For this review, take the finished solid that the model builds, in its own axes (mm). A direction names the side the tool comes from. Give positions to 0.01 mm unless a question says otherwise; leave off trailing zeros. Order: outer loops, then holes, each group sorted by start corner. A loop starts at its lowest first (then second) coordinate and runs counter-clockwise, first axis right, second up. Notation, with made-up numbers: (76, 13) -> (115, 13) arc R19 ccw to (115, 31) -> close; hole circle Ø4 at (30.25, -6). An arc over 180 degrees is marked (long way). Use CSV: the item, a comma, the result in double quotes. Start each with the question number.
```python
from build123d import *

# Parameters (mm, degrees)
SKETCH2_R          = 3.96875
CUT_EXTRUDE1_DEPTH = 6.35
CUT_EXTRUDE2_START = -41.402
CUT_EXTRUDE2_DEPTH = 31.75
SKETCH3_4_R        = 14.605
CUT_EXTRUDE3_DEPTH = 9.652


with BuildPart() as part:
    # Sketch1 → Revolve1 (revolve)
    with BuildSketch(Plane(origin=(0, 0, 0), x_dir=(1, 0, 0), z_dir=(0, 1, 0))):
        Polygon((-20.701, -12.7), (-20.701, -29.845), (-13.081, -29.845), (-13.081, -32.385), (5.969, -32.385), (5.969, -40.005), (7.239, -40.005), (7.239, -23.495), (20.701, -23.495), (20.701, -12.7), align=None)
    revolve(axis=Axis((-34.012862719, 0, 0), (1, 0, 0)))

    # Sketch2 → Cut-Extrude1 (cut)
    with BuildSketch(Plane(origin=(-20.701, 0, 0), x_dir=(0, 0, -1), z_dir=(1, 0, 0))):
        with Locations((22.225, 0)):
            Circle(SKETCH2_R)
        with Locations((-11.1125, -19.247414599)):
            Circle(SKETCH2_R)
        with Locations((-11.1125, 19.247414599)):
            Circle(SKETCH2_R)
    extrude(amount=CUT_EXTRUDE1_DEPTH, mode=Mode.SUBTRACT)

    # Sketch3 → Cut-Extrude2 (cut)
    with BuildSketch(Plane(origin=(20.701, 0, 0), x_dir=(0, 0, -1), z_dir=(1, 0, 0)).offset(CUT_EXTRUDE2_START)):
        with BuildLine():
            Line((-13.214999101, -6.218506553), (-10.722964654, -6.805000296))
            ThreePointArc((-10.722964654, -6.805000296), (-11.491303566, -5.407397003), (-12.078417757, -3.924515829))
            Line((-12.078417757, -3.924515829), (-13.214999101, -6.218506553))
        make_face()
        with BuildLine():
            Line((-14.346305297, -2.7367041), (-12.078417757, -3.924515829))
            ThreePointArc((-12.078417757, -3.924515829), (-12.475048084, -2.379742695), (-12.674939451, -0.797439598))
            Line((-12.674939451, -0.797439598), (-14.346305297, -2.7367041))
        make_face()
        with BuildLine():
            Line((-14.576180369, 0.917055538), (-12.674939451, -0.797439598))
            ThreePointArc((-12.674939451, -0.797439598), (-12.674939451, 0.797439598), (-12.475048084, 2.379742695))
            Line((-12.475048084, 2.379742695), (-14.576180369, 0.917055538))
        make_face()
        with BuildLine():
            Line((-13.89018042, 4.513193203), (-12.475048084, 2.379742695))
            ThreePointArc((-12.475048084, 2.379742695), (-12.078417757, 3.924515829), (-11.491303566, 5.407397003))
            Line((-11.491303566, 5.407397003), (-13.89018042, 4.513193203))
        make_face()
        with BuildLine():
            Line((-12.331409352, 7.825750341), (-11.491303566, 5.407397003))
            ThreePointArc((-11.491303566, 5.407397003), (-10.722964654, 6.805000296), (-9.785518183, 8.09528467))
            Line((-9.785518183, 8.09528467), (-12.331409352, 7.825750341))
        make_face()
        with BuildLine():
            Line((-9.997810482, 10.646586803), (-9.785518183, 8.09528467))
            ThreePointArc((-9.785518183, 8.09528467), (-8.693748245, 9.257901568), (-7.464872704, 10.274515829))
            Line((-7.464872704, 10.274515829), (-9.997810482, 10.646586803))
        make_face()
        with BuildLine():
            Line((-7.03601241, 12.798459062), (-7.464872704, 10.274515829))
            ThreePointArc((-7.464872704, 10.274515829), (-6.118271661, 11.129094837), (-4.675181819, 11.808161371))
            Line((-4.675181819, 11.808161371), (-7.03601241, 12.798459062))
        make_face()
        with BuildLine():
            Line((-3.632115802, 14.146157068), (-4.675181819, 11.808161371))
            ThreePointArc((-4.675181819, 11.808161371), (-3.158361567, 12.301006146), (-1.591732066, 12.599856707))
            Line((-1.591732066, 12.599856707), (-3.632115802, 14.146157068))
        make_face()
        with BuildLine():
            ThreePointArc((-1.591732066, 12.599856707), (0, 12.7), (1.591732066, 12.599856707))
            Line((1.591732066, 12.599856707), (0, 14.605))
            Line((0, 14.605), (-1.591732066, 12.599856707))
        make_face()
        with BuildLine():
            ThreePointArc((1.591732066, 12.599856707), (3.158361567, 12.301006146), (4.675181819, 11.808161371))
            Line((4.675181819, 11.808161371), (3.632115802, 14.146157068))
            Line((3.632115802, 14.146157068), (1.591732066, 12.599856707))
        make_face()
        with BuildLine():
            ThreePointArc((4.675181819, 11.808161371), (6.118271661, 11.129094837), (7.464872704, 10.274515829))
            Line((7.464872704, 10.274515829), (7.03601241, 12.798459062))
            Line((7.03601241, 12.798459062), (4.675181819, 11.808161371))
        make_face()
        with BuildLine():
            ThreePointArc((7.464872704, 10.274515829), (8.693748245, 9.257901568), (9.785518183, 8.09528467))
            Line((9.785518183, 8.09528467), (9.997810482, 10.646586803))
            Line((9.997810482, 10.646586803), (7.464872704, 10.274515829))
        make_face()
        with BuildLine():
            ThreePointArc((9.785518183, 8.09528467), (10.722964654, 6.805000296), (11.491303566, 5.407397003))
            Line((11.491303566, 5.407397003), (12.331409352, 7.825750341))
            Line((12.331409352, 7.825750341), (9.785518183, 8.09528467))
        make_face()
        with BuildLine():
            ThreePointArc((11.491303566, 5.407397003), (12.078417757, 3.924515829), (12.475048084, 2.379742695))
            Line((12.475048084, 2.379742695), (13.89018042, 4.513193203))
            Line((13.89018042, 4.513193203), (11.491303566, 5.407397003))
        make_face()
        with BuildLine():
            ThreePointArc((12.7, 0), (12.693733317, -0.39891664), (12.674939451, -0.797439598))
            Line((12.674939451, -0.797439598), (14.576180369, 0.917055538))
            Line((14.576180369, 0.917055538), (12.475048084, 2.379742695))
            ThreePointArc((12.475048084, 2.379742695), (12.64363695, 1.195175579), (12.7, 0))
        make_face()
        with BuildLine():
            ThreePointArc((12.674939451, -0.797439598), (12.475048084, -2.379742695), (12.078417757, -3.924515829))
            Line((12.078417757, -3.924515829), (14.346305297, -2.7367041))
            Line((14.346305297, -2.7367041), (12.674939451, -0.797439598))
        make_face()
        with BuildLine():
            ThreePointArc((12.078417757, -3.924515829), (11.491303566, -5.407397003), (10.722964654, -6.805000296))
            Line((10.722964654, -6.805000296), (13.214999101, -6.218506553))
            Line((13.214999101, -6.218506553), (12.078417757, -3.924515829))
        make_face()
        with BuildLine():
            ThreePointArc((10.722964654, -6.805000296), (9.785518183, -8.09528467), (8.693748245, -9.257901568))
            Line((8.693748245, -9.257901568), (11.253345911, -9.30957737))
            Line((11.253345911, -9.30957737), (10.722964654, -6.805000296))
        make_face()
        with BuildLine():
            ThreePointArc((8.693748245, -9.257901568), (7.464872704, -10.274515829), (6.118271661, -11.129094837))
            Line((6.118271661, -11.129094837), (8.58460361, -11.815693203))
            Line((8.58460361, -11.815693203), (8.693748245, -9.257901568))
        make_face()
        with BuildLine():
            Line((1.830491876, -14.489835213), (3.158361567, -12.301006146))
            ThreePointArc((3.158361567, -12.301006146), (1.591732066, -12.599856707), (0, -12.7))
            Line((0, -12.7), (1.830491876, -14.489835213))
        make_face()
        with BuildLine():
            Line((-1.830491876, -14.489835213), (0, -12.7))
            ThreePointArc((0, -12.7), (-1.591732066, -12.599856707), (-3.158361567, -12.301006146))
            Line((-3.158361567, -12.301006146), (-1.830491876, -14.489835213))
        make_face()
        with BuildLine():
            Line((-5.376459092, -13.579385576), (-3.158361567, -12.301006146))
            ThreePointArc((-3.158361567, -12.301006146), (-4.675181819, -11.808161371), (-6.118271661, -11.129094837))
            Line((-6.118271661, -11.129094837), (-5.376459092, -13.579385576))
        make_face()
        with BuildLine():
            Line((-8.58460361, -11.815693203), (-6.118271661, -11.129094837))
            ThreePointArc((-6.118271661, -11.129094837), (-7.464872704, -10.274515829), (-8.693748245, -9.257901568))
            Line((-8.693748245, -9.257901568), (-8.58460361, -11.815693203))
        make_face()
        with BuildLine():
            Line((-11.253345911, -9.30957737), (-8.693748245, -9.257901568))
            ThreePointArc((-8.693748245, -9.257901568), (-9.785518183, -8.09528467), (-10.722964654, -6.805000296))
            Line((-10.722964654, -6.805000296), (-11.253345911, -9.30957737))
        make_face()
        with BuildLine():
            Line((6.118271661, -11.129094837), (5.376459092, -13.579385576))
            Line((5.376459092, -13.579385576), (3.158361567, -12.301006146))
            ThreePointArc((3.158361567, -12.301006146), (4.675181819, -11.808161371), (6.118271661, -11.129094837))
        make_face()
    extrude(amount=CUT_EXTRUDE2_DEPTH, mode=Mode.SUBTRACT)

    # Sketch3<4> → Cut-Extrude3 (cut)
    with BuildSketch(Plane(origin=(20.701, 0, 0), x_dir=(0, 0, -1), z_dir=(1, 0, 0))):
        Circle(SKETCH3_4_R)
    extrude(amount=-CUT_EXTRUDE3_DEPTH, mode=Mode.SUBTRACT)


solid = part.part
```
1. To check wall thickness, follow L1, parallel to Y at x = 15, z = 0 (3 decimals); L2, parallel to Y at x = -15.5, z = -13; L3, parallel to Y at x = -17, z = 8.5. State the ranges of each line that lie inside material, in increasing order. Write a range as [from, to].
2. Consider section D-D (y = -26). State the section outline as (x, z) points, plus the area to 3 significant figures.
3. For faces 1 (the face through (-5.048, 13.362, 2.598)), 2 (the face through (11.049, 13, -5)), 3 (the face through (-17.57, 0.17, -18.26)), list the 3-axis set-ups (+Z, -Z, +X, -X, +Y, -Y) from which the entire face can be reached by the end or side of a thin tool; tool diameter is ignored.
4. Consider section B-B (y = 26.5). State the section outline as (x, z) points, plus the area to 3 significant figures.
5. Clearance check with flat-ended pins moving along their axes: P1, Ø3, axis at y = -10, z = -9.5, coming from the +X side; P2, Ø1, axis at x = 3, z = -9.5, coming from the -Y side; P3, Ø1, axis at x = -14, z = -20.5, coming from the +Y side; P4, Ø1, axis at x = -9.5, y = -8.5, coming from the +Z side. State where each tip first meets the part, or that it passes through.
6. Consider section A-A (x = 17.5). State the section outline as (y, z) points (3 decimals), plus the area to 3 significant figures.
7. Consider section C-C (z = -24.5). State the section outline as (x, y) points.
8. Draft analysis for pull direction Y (two halves, no side actions). For faces 4 (the face through (-13.081, 9, -29)), 5 (the face through (-17.57, -16.57, 14.04)), state which applies: +Y half, -Y half, draft (parallel to the pull), parting line (faces both ways), or undercut.
Answer list:
1,L1,"[-23.495, -14.605], [14.605, 23.495]"
1,L2,"[-26.86, -6.27], [-5.78, -3.44], [-1.17, -0.5], [2.01, 3.17], [4.85, 26.86]"
1,L3,"[-28.61, -22.24], [-16.26, -11.79], [10.43, 16.26], [22.24, 28.61]"
2,outline,"(-20.7, -14.65) -> (-13.08, -14.65) -> (-13.08, -19.31) -> (5.97, -19.31) -> (5.97, -30.4) -> (7.24, -30.4) -> (7.24, 30.4) -> (5.97, 30.4) -> (5.97, 19.31) -> (-13.08, 19.31) -> (-13.08, 14.65) -> (-20.7, 14.65) -> close"
2,area,"1,040 mm2"
3,face 1,"+X, -X"
3,face 2,"+X"
3,face 3,"-X"
4,outline,"(-20.7, -13.73) -> (-13.08, -13.73) -> (-13.08, -18.62) -> (5.97, -18.62) -> (5.97, -29.97) -> (7.24, -29.97) -> (7.24, 29.97) -> (5.97, 29.97) -> (5.97, 18.62) -> (-13.08, 18.62) -> (-13.08, 13.73) -> (-20.7, 13.73) -> close"
4,area,"995 mm2"
5,P1,"x = 20.7"
5,P2,"y = -31.11"
5,P3,"y = 22.15"
5,P4,"z = 31.38"
6,outline,"circle Ø46.99 at (0, 0); hole circle Ø29.21 at (0, 0)"
6,area,"1,060 mm2"
7,outline,"(-20.7, -17.04) -> (-13.08, -17.04) -> (-13.08, -21.18) -> (5.97, -21.18) -> (5.97, -31.63) -> (7.24, -31.63) -> (7.24, 31.63) -> (5.97, 31.63) -> (5.97, 21.18) -> (-13.08, 21.18) -> (-13.08, 17.04) -> (-20.7, 17.04) -> (-20.7, 3.25) -> (-14.35, 3.25) -> (-14.35, -3.25) -> (-20.7, -3.25) -> close"
8,face 4,"draft"
8,face 5,"undercut"
